Source: CAD feature listing. Evaluate the final solid. Frame: model axes, mm. Coordinates: 2 decimals unless noted, no trailing zeros. Order: outer loops, then holes, each group sorted by start corner. A loop starts at its lowest first (then second) coordinate and runs counter-clockwise, first axis right, second up. Notation, with made-up numbers: (10, -9) - (52, -9) arc R15 cw to (52, -2) - close; hole circle Ø3 at (4.25, 49.25). An arc over 180 degrees is marked (long way). One line per question, with ' | ' between items. Start each with the question number.
(1) Section B-B (z = 94). Return the cut outline in (x, y) (1 decimal), then the cut area to 3 significant figures.
(2) Contact query for flat-ended pins moving along their axis: P1, Ø2.5, axis at x = -0.5, z = 3.5, coming from the +Y side; P2, Ø2, axis at x = 9.5, y = -7, coming from the +Z side; P3, Ø0.8, axis at x = 0, y = 3, coming from the -Z side. Output: stop coordinate, or through.
(3) Section C-C (x = 9.5). Return the cut outline in (y, z).
(4) Section A-A (z = 7). Return the cut outline in (x, y) (1 decimal).
(5) Line query: line 1 along Y through (x, z) = (5, 6.5); line 2 along X through (y, z) = (3.75, 10) (3 decimals); line 3 along Z through (x, y) = (-4.5, -2.5). Output: solid intervals per line, ascending.
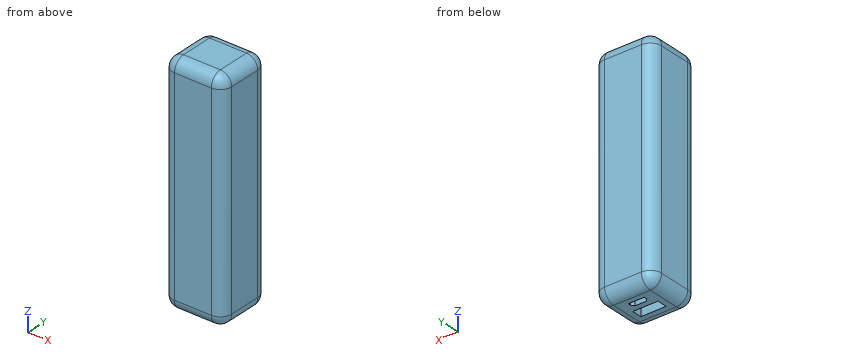
Autodesk Inventor part; units mm, degrees
ref_plane "YZ Plane" through (0, 0, 0) normal (1, 0, 0) x (0, 1, 0)
ref_plane "XZ Plane" through (0, 0, 0) normal (0, 1, 0) x (-1, 0, 0)
ref_plane "XY Plane" through (0, 0, 0) normal (0, 0, 1) x (1, 0, 0)
sketch "Sketch1" plane through (0, 0, 0) normal (0, 0, 1) x (1, 0, 0)
  line L0 (-13.335, 12.3825) -> (13.335, 12.3825)
  line L1 (13.335, 12.3825) -> (13.335, -12.3825)
  line L2 (13.335, -12.3825) -> (-13.335, -12.3825)
  line L3 (-13.335, -12.3825) -> (-13.335, 12.3825)
  line L4 (-13.335, 12.3825) -> (13.335, -12.3825) construction
  line L5 (13.335, 12.3825) -> (-13.335, -12.3825) construction
  point P0 (0, 0)
  dimension "d0" = 26.67
  dimension "d1" = 24.765
extrude "Extrusion1" add sketch "Sketch1" along normal blind 102.87
fillet "Fillet1" radius 5.08 12 edges at (13.335, 12.3825, 51.435) (13.335, 0, 102.87) (0, 12.3825, 102.87) (0, -12.3825, 102.87) (13.335, -12.3825, 51.435) (-13.335, 0, 102.87) (13.335, 0, 0) (0, 12.3825, 0) (-13.335, 0, 0) (0, -12.3825, 0) (-13.335, 12.3825, 51.435) (-13.335, -12.3825, 51.435)
sketch "Sketch2" plane through (0, 0, 0) normal (0, 0, -1) x (-1, 0, 0)
  line L0 (-5.715, -0.1905) -> (5.715, -0.1905)
  line L1 (5.715, -0.1905) -> (5.715, -4.7625)
  line L2 (5.715, -4.7625) -> (-5.715, -4.7625)
  line L3 (-5.715, -4.7625) -> (-5.715, -0.1905)
  line L4 (-8.255, -12.3825) -> (8.255, -12.3825)
  line L5 (-8.255, 12.3825) -> (8.255, 12.3825) construction
  line L6 (0, 12.3825) -> (0, -12.3825) construction
  line L7 (-3.556, 4.8895) -> (3.556, 4.8895)
  line L8 (3.556, 4.8895) -> (3.556, 3.6195)
  line L9 (-3.556, 4.8895) -> (-3.556, 3.6195)
  line L10 (-2.54, 2.3495) -> (2.54, 2.3495)
  line L11 (2.54, 2.3495) -> (3.556, 3.6195)
  line L12 (-3.556, 3.6195) -> (-2.54, 2.3495)
  point P0 (0, 0)
  dimension "d5" = 11.43
  dimension "d6" = 4.572
  dimension "d7" = 7.62
  dimension "d8" = 5.715
  dimension "d9" = 7.112
  dimension "d10" = 1.27
  dimension "d11" = 1.27
  dimension "d12" = 5.08
  dimension "d13" = 2.54
  dimension "d14" = 1.016
  dimension "d15" = 3.556
  dimension "d16" = 2.54
extrude "Extrusion2" cut sketch "Sketch2" against normal blind 12.7
equation "\"d8\" = 0.5 * d5"
equation "\"d15\" = 0.5 * d9"
properties part number "5V_LIon"
Response values:
1) outline: (-13.3, -7.3) arc R5.1 ccw to (-8.3, -12.4) - (8.3, -12.4) arc R5.1 ccw to (13.3, -7.3) - (13.3, 7.3) arc R5.1 ccw to (8.3, 12.4) - (-8.3, 12.4) arc R5.1 ccw to (-13.3, 7.3) - close | area: 638 mm²
2) P1: stops at y = 12.37 | P2: stops at z = 102.86 | P3: stops at z = 12.7
3) outline: (-12.23, 5.08) arc R4.93 ccw to (-7.3, 0.15) - (7.3, 0.15) arc R4.93 ccw to (12.23, 5.08) - (12.23, 97.79) arc R4.93 ccw to (7.3, 102.72) - (-7.3, 102.72) arc R4.93 ccw to (-12.23, 97.79) - close
4) outline: (-13.3, -7.3) arc R5.1 ccw to (-8.3, -12.4) - (8.3, -12.4) arc R5.1 ccw to (13.3, -7.3) - (13.3, 7.3) arc R5.1 ccw to (8.3, 12.4) - (-8.3, 12.4) arc R5.1 ccw to (-13.3, 7.3) - close; hole (-5.7, -4.8) - (5.7, -4.8) - (5.7, -0.2) - (-5.7, -0.2) - close; hole (-3.6, 3.6) - (-2.5, 2.3) - (2.5, 2.3) - (3.6, 3.6) - (3.6, 4.9) - (-3.6, 4.9) - close
5) line 1: y = -12.38 to -4.76, -0.19 to 12.38 | line 2: x = -13.335 to -3.556, 3.556 to 13.335 | line 3: z = 12.7 to 102.87
